Geometry check sheet. Reference: drawing and pictorial views, mm from the part's lowest x, y, z. A direction names the side the tool comes from. Give positions to 0.01 mm unless a question says otherwise; leave off trailing zeros. Write each loop counter-clockwise with the first axis right and the second up, starting at its lowest first coordinate (ties: lowest second). Pieces come first, ordered by that corner, then holes. Notation, with made-up numbers: M 87.25,-32 L 115.25,-32 A30 ccw 115.25,-8 Z; hole C 44.25,-35.75 d10. An arc over 180 degrees is marked long. Write item = value, one per line. Start each with the question number.
1) Cross-section at B-B, the plane z = 6. Record the cut outline in (x, y).
2) Scan lines: line 1 along X through (y, z) = (22.5, 0.5); line 2 along Z through (x, y) = (15.75, 12); line 3 along Y through (x, z) = (5.5, 6). Record each from-to range of solid material in increasing order. Write a range as [from, to].
3) Access from +Z, -Z, +X, -X, +Y, -Y to the whole of each face (thin tool, end or side, straight path). Record for the marked faces 4, 5 and 6.
4) Cross-section at D-D, the plane x = 18.25. Record the cut outline in (y, z).
5) Cross-section at C-C, the plane z = 3. Record the cut outline in (x, y), plus the area to 3 significant figures.
6) Cross-section at A-A, the plane y = 16. Record the cut outline in (x, z).
7) Go/stop test with flat-tipped pins: pin 1 (8 mm diameter, centred on x = 15, y = 12, fed in from +Z); pin 2 (0.9 mm diameter, centred on x = 22, z = 4.5, fed in from -Y). Record where each tip stops, or that it passes through.
8) Mould release check, pull along X, two halves, no side actions. Record for the marked faces 1, 2 and 3: released by +X, released by -X, zero draft, split by the parting line, or undercut.
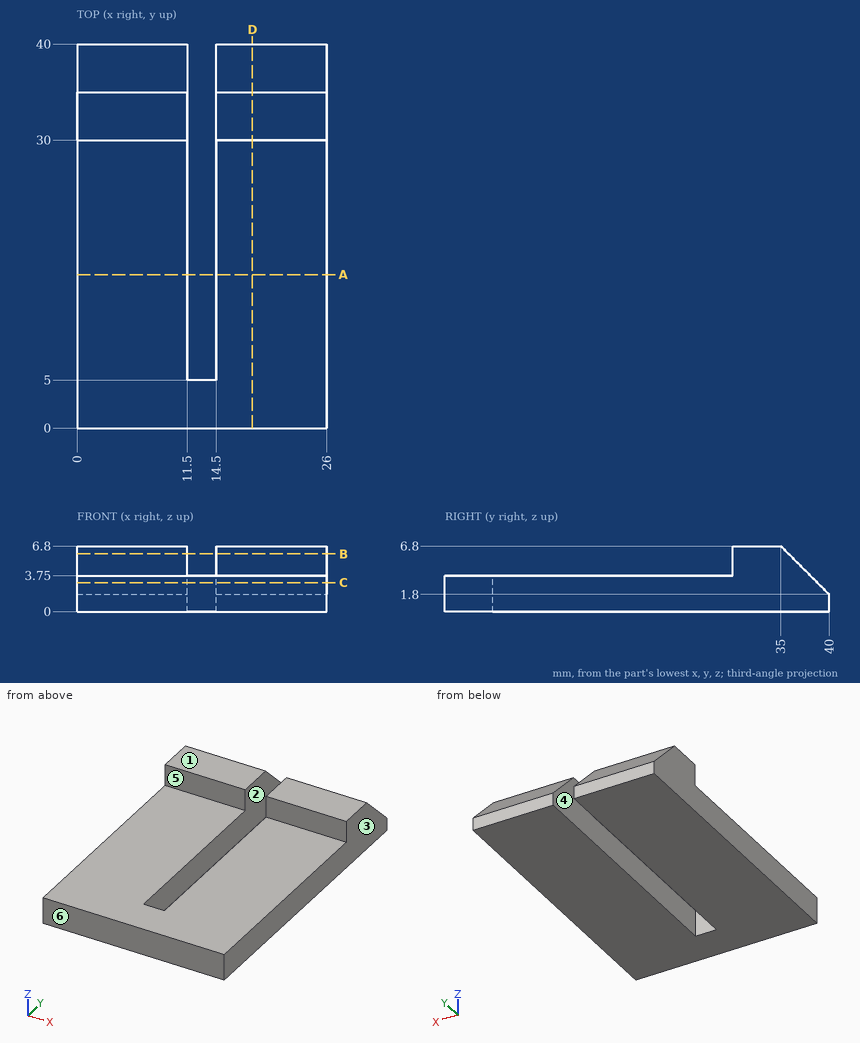
Reply:
q1.outline = M 0,30 L 11.5,30 L 11.5,35.8 L 0,35.8 Z; M 14.5,30 L 26,30 L 26,35.8 L 14.5,35.8 Z
q2.line_1 = [0, 11.5], [14.5, 26]
q2.line_2 = [0, 3.75]
q2.line_3 = [30, 35.8]
q3.face_4 = +Z, -Z, +Y
q3.face_5 = +Z, +X, -X, -Y
q3.face_6 = +Z, -Z, +X, -X, -Y
q4.outline = M 0,0 L 40,0 L 40,1.8 L 35,6.8 L 30,6.8 L 30,3.75 L 0,3.75 Z
q5.outline = M 0,0 L 26,0 L 26,38.8 L 14.5,38.8 L 14.5,5 L 11.5,5 L 11.5,38.8 L 0,38.8 Z
q5.area = 907 mm2
q6.outline = M 0,0 L 11.5,0 L 11.5,3.75 L 0,3.75 Z; M 14.5,0 L 26,0 L 26,3.75 L 14.5,3.75 Z
q7.pin_1 = 3.75
q7.pin_2 = 30
q8.face_1 = zero draft
q8.face_2 = undercut
q8.face_3 = released by +X
